The model under review builds one solid part; all positions refer to its coordinate system, in mm. Face numbers are marked on the shaded views. A direction names the side the tool comes from. Coordinates: 2 decimals unless noted, no trailing zeros. Loops run counter-clockwise (first coordinate to the right, second up) from the corner with the lowest first, then second, coordinate; pieces in that order, holes last. Notation, with made-up numbers: M -2.5,-10.75 L 32.5,-10.75 A28 ccw 32.5,16.25 Z; hole C -15.75,59 d4. An arc over 180 degrees is marked long. Use CSV: the item, a comma, the result in double quotes. Start each with the question number.
from build123d import *

# Parameters (mm, degrees)
F0_W     = 87.010126
F0_H     = 52.755846
F0_W_2   = 81.010126
F0_H_2   = 46.755846
F1_DEPTH = 27.94
F0_R     = 7.07637
F0_R_2   = 6.824526
F0_R_3   = 7.16417
F0_R_4   = 6.915523
F2_DEPTH = 5.842


with BuildPart() as f1:
    # F0 (on Top) → F1 (new body)
    with BuildSketch(Plane.XY):
        Rectangle(F0_W, F0_H)
        Rectangle(F0_W_2, F0_H_2, mode=Mode.SUBTRACT)
    extrude(amount=F1_DEPTH)

    # F0 (on Top) → F2 (join)
    with BuildSketch(Plane.XY):
        Rectangle(F0_W, F0_H)
        Rectangle(F0_W_2, F0_H_2, mode=Mode.SUBTRACT)
        Rectangle(F0_W_2, F0_H_2)
        with Locations((-27.253406, -13.626703)):
            Circle(F0_R, mode=Mode.SUBTRACT)
        with Locations((27.253406, -13.626703)):
            Circle(F0_R_2, mode=Mode.SUBTRACT)
        with Locations((-27.253406, 13.626703)):
            Circle(F0_R_3, mode=Mode.SUBTRACT)
        with Locations((27.253406, 13.626703)):
            Circle(F0_R_4, mode=Mode.SUBTRACT)
    extrude(amount=F2_DEPTH)


solid = f1.part
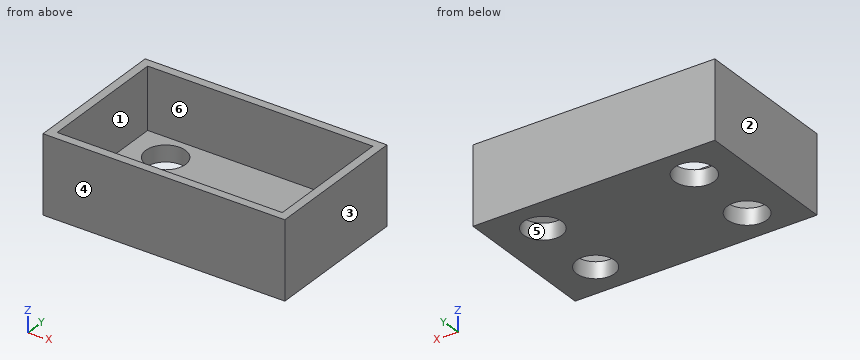
1. Add section B-B (y = 4.5). Write out the cut boundary in (x, z).
2. For the marked faces 1 and 2, list the 3-axis set-ups (+Z, -Z, +X, -X, +Y, -Y) from which the entire face can be reached by the end or side of a thin tool; tool diameter is ignored.
3. Add section A-A (z = 7.5). Write out the cut boundary in (x, y), plus the area to 3 significant figures.
4. Add section C-C (x = -30). Write out the cut boundary in (y, z), plus the area to 3 significant figures.
5. Draft analysis for pull direction X (two halves, no side actions). For the marked faces 3, 4, 5 and 6, state which applies: released by +X, released by -X, zero draft, split by the parting line, or undercut.
6. Add section D-D (y = 19). Write out the cut boundary in (x, z), plus the area to 3 significant figures.
7. Insertion check: pin 1 Ø12.5 at (x, y) = (27.25, 13.63) entering from -Z; pin 2 Ø8 at (x, y) = (5.5, -12.5) entering from +Z. Each pin has a flat end and moves straight along its axis. Give the tip position at first contact, or say it passes through.
8. To check wall thickness, follow line 1 along Y through (x, z) = (-13, 22.5); line 2 along X through (y, z) = (15, 14.75); line 3 along X through (y, z) = (8, 4). State the ranges of each line that lie inside material, in increasing order.
Solved:
1,outline,"M -43.51,0 L 43.51,0 L 43.51,27.94 L 40.51,27.94 L 40.51,5.84 L -40.51,5.84 L -40.51,27.94 L -43.51,27.94 Z"
2,face 1,"+Z"
2,face 2,"+Z, -Z, -X, +Y, -Y"
3,outline,"M -43.51,-26.38 L 43.51,-26.38 L 43.51,26.38 L -43.51,26.38 Z; hole M -40.51,-23.38 L 40.51,-23.38 L 40.51,23.38 L -40.51,23.38 Z"
3,area,"803 mm^2"
4,outline,"M -26.38,0 L -20.15,0 L -20.15,5.84 L -23.38,5.84 L -23.38,27.94 L -26.38,27.94 Z; M -7.11,0 L 7.01,0 L 7.01,5.84 L -7.11,5.84 Z; M 20.24,0 L 26.38,0 L 26.38,27.94 L 23.38,27.94 L 23.38,5.84 L 20.24,5.84 Z"
4,area,"287 mm^2"
5,face 3,"released by +X"
5,face 4,"zero draft"
5,face 5,"undercut"
5,face 6,"undercut"
6,outline,"M -43.51,0 L -31.99,0 L -31.99,5.84 L -40.51,5.84 L -40.51,27.94 L -43.51,27.94 Z; M -22.51,0 L 22.9,0 L 22.9,5.84 L -22.51,5.84 Z; M 31.61,0 L 43.51,0 L 43.51,27.94 L 40.51,27.94 L 40.51,5.84 L 31.61,5.84 Z"
6,area,"535 mm^2"
7,pin 1,"passes through"
7,pin 2,"stops at z = 5.84"
8,line 1,"y = -26.38 to -23.38, 23.38 to 26.38"
8,line 2,"x = -43.51 to -40.51, 40.51 to 43.51"
8,line 3,"x = -43.51 to -31.69, -22.82 to 23.23, 31.27 to 43.51"
